Source: CAD feature listing. Evaluate the final solid. Frame: model axes, mm. Face numbers are marked on the shaded views. Give positions to 0.01 mm unless a question says otherwise; leave off trailing zeros. Order: outer loops, then holes, each group sorted by start corner. A loop starts at its lowest first (then second) coordinate and runs counter-clockwise, first axis right, second up. Notation, with made-up numbers: M 19,-6 L 29,-6 A11 cw 29,4 Z; hole C 70.25,-6 d11. An arc over 180 degrees is marked long. Answer in a Markdown table with one row per item. Add a question column.
(1) Pin query (flat end, axial travel): P1, Ø8, axis at y = -6, z = 23, coming from the -X side; P2, Ø1, axis at x = 5.5, z = 24, coming from the -Y side; P3, Ø4, axis at x = -2.5, z = 24, coming from the +Y side. Return the tip coordinate at first contact, or that it passes through.
(2) Section query D-D, the plane x = 2.75. Return loops of the section in (y, z).
(3) Section query B-B, the plane z = 29.5. Return loops of the section in (x, y) (3 decimals), plus the area to 3 significant figures.
(4) Material intervals for line 1 along Y through (x, z) = (0, 15.5) (3 decimals); line 2 along Y through (x, z) = (-7.5, 21); line 3 along X through (y, z) = (4, 28), sorted ascending.
(5) Section query A-A, the plane x = 0.75. Return loops of the section in (y, z).
(6) Mould query, pull axis X, two halves, no side actions, for the marked faces 1, 2 and 3. Classes: pulls with the +X half, pulls with the -X half, needs draft (parallel to the pull), parting line crosses it, or undercut.
(7) Section query C-C, the plane y = -6.75. Return loops of the section in (x, z), plus the area to 3 significant figures.
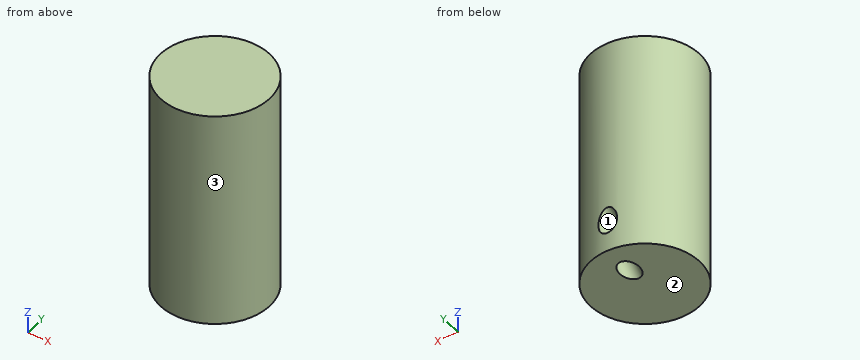
Autodesk Inventor part; units mm, degrees
ref_plane "Work Plane3" through (0, 9.525, 0) normal (0, 0.7071, 0.7071) x (-1, 0, 0)
ref_plane "YZ Plane" through (0, 0, 0) normal (1, 0, 0) x (0, 1, 0)
ref_plane "XY Plane" through (0, 0, 0) normal (0, 0, 1) x (1, 0, 0)
sketch "Sketch1" plane through (0, 0, 0) normal (0, 0, 1) x (1, 0, 0)
  circle A0 centre (0, 0) radius 9.525
  dimension "d0" = 19.05
extrude "Extrusion1" add sketch "Sketch1" along normal blind 38.1
ref_plane "Work Plane2" through (0, 15.875, 0) normal (0, 1, 0) x (-1, 0, 0)
sketch "Sketch4" plane through (0, 15.875, 0) normal (0, 1, 0) x (-1, 0, 0)
  circle A0 centre (0, 7.62) radius 1.4605
  point P0 (0, 0)
  dimension "d6" = 2.921
  dimension "d7" = 7.62
sketch "Sketch5" plane through (0, 0, 0) normal (0, 0, -1) x (-1, 0, 0)
  circle A0 centre (0, 0) radius 9.525
  circle A1 centre (0, 1.905) radius 1.4605
  line L0 (0, 9.525) -> (14.2875, 9.525)
  dimension "d8" = 2.921
  dimension "d9" = 7.62
ref_plane "Work Plane3" through (0, 9.525, 0) normal (0, 0.7071, 0.7071) x (-1, 0, 0)
sketch "Sketch6" plane through (0, 9.525, 0) normal (0, 0.7071, 0.7071) x (-1, 0, 0)
  circle A0 centre (0, 3.9683) radius 1.5875
  point P0 (0, 6.7352)
  dimension "d11" = 3.175
extrude "Extrusion2" add sketch "Sketch6" along normal mid plane 25.4
sketch "Sketch7" plane through (0, -2.2613, -6.1742) normal (0, -0.7071, -0.7071) x (-1, 0, 0)
  circle A0 centre (0, 0) radius 1.5875
  circle A1 centre (0, 0) radius 1.5875
  point P0 (0, -2.7669)
hole "Hole1" at (-0.0004, -2.2603, -6.1752) direction (0, 0.7071, 0.7071) diameter 3.302 depth 25.4 tip angle 118
properties part number "Brass"
Values follow:
| question | item | result |
|---|---|---|
| 1 | P1 | stops at x = -9.31 |
| 1 | P2 | stops at y = -8.11 |
| 1 | P3 | stops at y = 9.51 |
| 2 | outline | M -9.12,0 L 9.12,0 L 9.12,38.1 L -9.12,38.1 Z |
| 3 | outline | C 0,0 d19.05 |
| 3 | area | 285 mm² |
| 4 | line 1 | y = -9.525 to 9.525 |
| 4 | line 2 | y = -5.87 to 5.87 |
| 4 | line 3 | x = -8.64 to 8.64 |
| 5 | outline | M -9.5,0 L 1.84,0 L 9.5,7.66 L 9.5,38.1 L -9.5,38.1 Z; M 5.99,0 L 9.5,0 L 9.5,3.5 Z |
| 6 | face 1 | undercut |
| 6 | face 2 | needs draft |
| 6 | face 3 | parting line crosses it |
| 7 | outline | M -6.72,0 L 6.72,0 L 6.72,38.1 L -6.72,38.1 Z |
| 7 | area | 512 mm² |
